Here's how the part is built. I have some questions about the finished solid (model axes, mm). A direction names the side the tool comes from. Give positions to 0.01 mm unless a question says otherwise; leave off trailing zeros. Write each loop counter-clockwise with the first axis right and the second up, starting at its lowest first coordinate (ties: lowest second). Pieces come first, ordered by that corner, then holes. Notation, with made-up numbers: (59, 18) -> (79, 18) arc R7 ccw to (79, 22) -> close; hole circle Ø6 at (-19, 72.5). An arc over 180 degrees is marked (long way). Return JSON: item names as keys, results as strings.
from build123d import *

# Parameters (mm, degrees)
SKETCH1_R                 = 3
BOSS_EXTRUDE1_DEPTH       = 29
SKETCH2_R                 = 6
BOSS_EXTRUDE2_DEPTH       = 2.1
SKETCH3_R                 = 12.7
BOSS_EXTRUDE3_DEPTH       = 5
SKETCH4_R                 = 6
BOSS_EXTRUDE4_DEPTH       = 2.1
F_4_40_TAPPED_HOLE1_D     = 2.2606
F_4_40_TAPPED_HOLE1_DEPTH = 7.6
F_4_40_TAPPED_HOLE1_TIP   = 0.679152758


with BuildPart() as part:
    # Sketch1 → Boss-Extrude1 (new body)
    with BuildSketch(Plane.XY):
        Circle(SKETCH1_R)
    extrude(amount=BOSS_EXTRUDE1_DEPTH)

    # Sketch2 → Boss-Extrude2 (add)
    with BuildSketch(Plane.XY.offset(8)):
        Circle(SKETCH2_R)
    extrude(amount=-BOSS_EXTRUDE2_DEPTH)

    # Sketch3 → Boss-Extrude3 (add)
    with BuildSketch(Plane(origin=(0, 0, 5.9), x_dir=(-1, 0, 0), z_dir=(0, 0, -1))):
        Circle(SKETCH3_R)
    extrude(amount=BOSS_EXTRUDE3_DEPTH)

    # Sketch4 → Boss-Extrude4 (add)
    with BuildSketch(Plane.XY.offset(8)):
        Circle(SKETCH4_R)
    extrude(amount=BOSS_EXTRUDE4_DEPTH)

    # #4-40 Tapped Hole1
    with Locations(Plane(origin=(0, 0, 0.9), x_dir=(-1, 0, 0), z_dir=(0, 0, -1))):
        with Locations((8.227241336, 4.75), (8.227241336, -4.75), (0, -9.5), (-8.227241336, -4.75), (-8.227241336, 4.75), (0, 9.5)):
            Hole(F_4_40_TAPPED_HOLE1_D / 2, depth=F_4_40_TAPPED_HOLE1_DEPTH)
            with Locations((0, 0, -(F_4_40_TAPPED_HOLE1_DEPTH + F_4_40_TAPPED_HOLE1_TIP / 2))):  # 118° drill point
                Cone(0, F_4_40_TAPPED_HOLE1_D / 2, F_4_40_TAPPED_HOLE1_TIP, mode=Mode.SUBTRACT)


solid = part.part
1. Suppose I cut it at B-B, the plane z = 2.5. List the corners of the cut face in (x, y) for me, and give its area (3 significant figures).
Taken from the geometry:
{"outline": "circle Ø25.4 at (0, 0); hole circle Ø2.26 at (-8.23, -4.75); hole circle Ø2.26 at (-8.23, 4.75); hole circle Ø2.26 at (0, -9.5); hole circle Ø2.26 at (0, 9.5); hole circle Ø2.26 at (8.23, -4.75); hole circle Ø2.26 at (8.23, 4.75)", "area": "483 mm²"}
2. If I drill on line 1 (Y direction, x = 0, z = 1.95); line 2 (Z direction, x = 8, y = -6); line 3 (Z direction, x = 2, y = -3), over which ranges is the centre line in solid material (lowest first)? Write a range as [from, to].
Taken from the geometry:
{"line 1": "y = [-12.7, -10.63], [-8.37, 8.37], [10.63, 12.7]", "line 2": "z = [0.9, 5.9]", "line 3": "z = [0.9, 10.1]"}
3. Suppose I cut it at D-D, the plane y = -4.75. List the corners of the cut face in (x, z) for me.
Taken from the geometry:
{"outline": "(-11.78, 0.9) -> (-9.36, 0.9) -> (-9.36, 5.9) -> (-11.78, 5.9) -> close; (-7.1, 0.9) -> (7.1, 0.9) -> (7.1, 5.9) -> (3.67, 5.9) -> (3.67, 10.1) -> (-3.67, 10.1) -> (-3.67, 5.9) -> (-7.1, 5.9) -> close; (9.36, 0.9) -> (11.78, 0.9) -> (11.78, 5.9) -> (9.36, 5.9) -> close"}
4. Suppose I cut it at C-C, the plane y = -10. List the corners of the cut face in (x, z) for me, and give its area (3 significant figures).
Taken from the geometry:
{"outline": "(-7.83, 0.9) -> (-1.01, 0.9) -> (-1.01, 5.9) -> (-7.83, 5.9) -> close; (1.01, 0.9) -> (7.83, 0.9) -> (7.83, 5.9) -> (1.01, 5.9) -> close", "area": "68.2 mm²"}
5. Suppose I cut it at A-A, the plane x = 0. List the corners of the cut face in (y, z) for me, and give its area (3 significant figures).
Taken from the geometry:
{"outline": "(-12.7, 0.9) -> (-10.63, 0.9) -> (-10.63, 5.9) -> (-12.7, 5.9) -> close; (-8.37, 0.9) -> (-3, 0.9) -> (-3, 0) -> (3, 0) -> (3, 0.9) -> (8.37, 0.9) -> (8.37, 5.9) -> (6, 5.9) -> (6, 10.1) -> (3, 10.1) -> (3, 29) -> (-3, 29) -> (-3, 10.1) -> (-6, 10.1) -> (-6, 5.9) -> (-8.37, 5.9) -> close; (10.63, 0.9) -> (12.7, 0.9) -> (12.7, 5.9) -> (10.63, 5.9) -> close", "area": "274 mm²"}
6. Which directions (+Z, -Z, +X, -X, +Y, -Y) give clear straight access to the entire face, cutting with the end or side of a thin tool? Please do faces 5 (the face through (0, 0, 0)), 6 (the face through (-3, -1, 10.1)), 7 (the face through (-3, -3, 0.9)).
Taken from the geometry:
{"face 5": "-Z, +X, -X, +Y, -Y", "face 6": "+Z", "face 7": "-Z"}
7. If we mould it in two halves opening along Y, with no side actions, what happens to faces 1 (the face through (7.982, -5.853, 3.435)), 2 (the face through (-0.15, 10.62, 3.44)), 3 (the face through (2.75, -12.4, 3.44)), 4 (the face through (3, -5.5, 5.9))? For each: released by +Y, released by -Y, zero draft, split by the parting line, or undercut.
Taken from the geometry:
{"face 1": "undercut", "face 2": "undercut", "face 3": "split by the parting line", "face 4": "zero draft"}
8. For pin 1 Ø1.4 at (x, y) = (-8.23, -4.75) entering from -Z; pin 2 Ø1 at (x, z) = (8.5, 6) entering from +Y; pin 3 Ø12 at (y, z) = (6, 24.5) entering from +X; pin 4 Ø3 at (x, y) = (0, -9.5) entering from +Z, each with a flat end and sliding along its axis, tell me the tip position at first contact or that it passes through.
Taken from the geometry:
{"pin 1": "passes through", "pin 2": "stops at y = 9.86", "pin 3": "stops at x = 3", "pin 4": "stops at z = 5.9"}
